The model under review builds one solid part; all positions refer to its coordinate system, in mm. A direction names the side the tool comes from. Coordinates: 2 decimals unless noted, no trailing zeros. Write each loop counter-clockwise with the first axis right and the second up, starting at its lowest first coordinate (ties: lowest second). Pieces come first, ordered by that corner, then holes.
Solid Edge part; units mm, degrees
sketch "Sketch1" plane through (0, 0, 0) normal (0, -1, 0) x (1, 0, 0)
  line L0 (-12, 28) -> (-7, 28)
  arc A0 (-7, 28) -> (0, 21) centre (0, 28) ccw
  arc A1 (7, 28) -> (0, 21) centre (0, 28) cw
  line L1 (12, 28) -> (7, 28)
  line L2 (12, 13) -> (12, 28)
  line L3 (14, 13) -> (12, 13)
  line L4 (14, 7) -> (14, 13)
  line L5 (0, 7) -> (14, 7)
  line L6 (0, 7) -> (-14, 7)
  line L7 (-14, 7) -> (-14, 13)
  line L8 (-14, 13) -> (-12, 13)
  line L9 (-12, 13) -> (-12, 28)
revolve "RevolvedProtrusion1" add sketch "Sketch1" angle 360 about axis through (0, 0, 0) along (1, 0, 0)
Item 1: Take a section at A-A, the plane y = 0. Write out the cut boundary in (x, z), plus the area to 3 significant figures.
Solved:
outline: (-14, -13) - (-12, -13) - (-12, -28) - (-7, -28) arc R7 cw to (7, -28) - (12, -28) - (12, -13) - (14, -13) - (14, -7) - (-14, -7) - close; (-14, 7) - (14, 7) - (14, 13) - (12, 13) - (12, 28) - (7, 28) arc R7 cw to (-7, 28) - (-12, 28) - (-12, 13) - (-14, 13) - close
area: 902 mm2
Item 2: To check wall thickness, follow line 1 along X through (y, z) = (19.5, 5); line 2 along Z through (x, y) = (-10.25, 3.5); line 3 along X through (y, z) = (-2, 21.5). State the ranges of each line that lie inside material, in increasing order.
Solved:
line 1: x = -12 to 12
line 2: z = -27.78 to -6.06, 6.06 to 27.78
line 3: x = -12 to -2.82, 2.82 to 12
Item 3: Take a section at C-C, the plane x = 1. Write out the cut boundary in (y, z), plus the area to 3 significant figures.
Solved:
outline: circle Ø42.14 at (0, 0); hole circle Ø14 at (0, 0)
area: 1,240 mm2
Item 4: For pin 1 (1 mm diameter, centred on x = -5.5, z = 16, fed in from +Y); pin 2 (10 mm diameter, centred on x = 1, y = -10.5, fed in from -Z); pin 3 (2 mm diameter, centred on y = -3.5, z = -18.5, fed in from -X), all flat-tipped, find the tip position at first contact; note any pin that passes through.
Solved:
pin 1: stops at y = 18.5
pin 2: stops at z = -22.3
pin 3: stops at x = -12
Item 5: Mouldability with a two-part tool opening along Z and no side actions: class faces 4 (the face through (0.196, 2.681, 6.466)), 5 (the face through (-9.465, 10.724, 25.865)), 6 (the face through (-14, 6, 6)) as pulls with the +Z half, pulls with the -Z half, needs draft (parallel to the pull), parting line crosses it, or undercut.
Solved:
face 4: undercut
face 5: parting line crosses it
face 6: needs draft
Item 6: Take a section at D-D, the plane x = -6.25. Write out the cut boundary in (y, z), plus the area to 3 significant figures.
Solved:
outline: circle Ø49.7 at (0, 0); hole circle Ø14 at (0, 0)
area: 1,790 mm2
Item 7: Machinability: for faces 1 (the face through (14, 6, 6)), 2 (the face through (-12.986, 7.91, -10.316)), 3 (the face through (12, 12, 6)), which of the approach directions +Z, -Z, +X, -X, +Y, -Y give a long, thin tool a straight path to every point of the face, cutting with its end or side? Answer none if there is none.
Solved:
face 1: +Z, -Z, +X, +Y, -Y
face 2: -X
face 3: +X
